Geometry check sheet. Reference: drawing and pictorial views, mm from the part's lowest x, y, z. A direction names the side the tool comes from. Give positions to 0.01 mm unless a question says otherwise; leave off trailing zeros. Write each loop counter-clockwise with the first axis right and the second up, starting at its lowest first coordinate (ties: lowest second). Pieces come first, ordered by that corner, then holes. Notation, with made-up numbers: (-0.75, 54.5) -> (51.25, 54.5) arc R3 cw to (51.25, 59.5) -> close; hole circle Ø2 at (12, -5). An arc over 180 degrees is marked (long way). Answer as CSV lines item,"result".
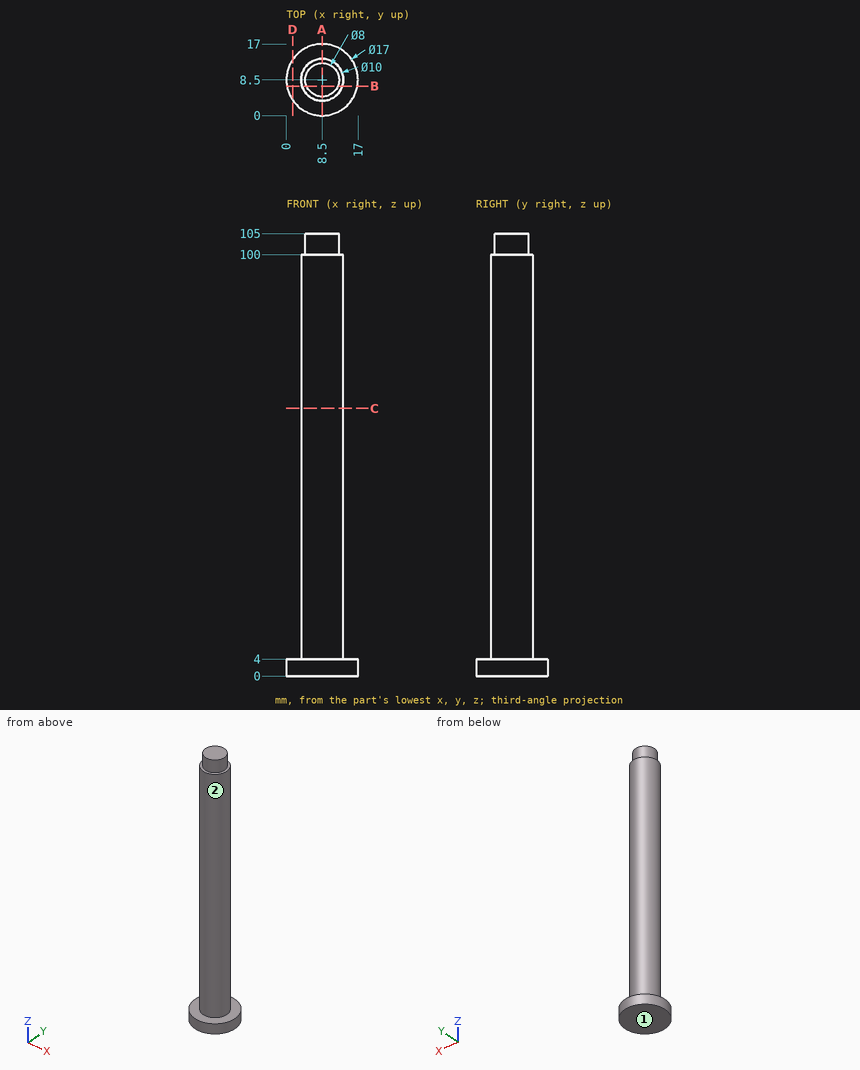
1) Section check C-C (z = 63.5). Record the boundary of the cut face in (x, y), and give its area (3 significant figures).
Reported:
outline,"circle Ø10 at (8.5, 8.5)"
area,"78.5 mm²"
2) Scan lines: line 1 along Y through (x, z) = (11.5, 61); line 2 along Y through (x, z) = (8.5, 78); line 3 along Z through (x, y) = (3, 6.25). Record each from-to range of solid material in increasing order.
Reported:
line 1,"4.5 to 12.5"
line 2,"3.5 to 13.5"
line 3,"0 to 4"
3) Section check D-D (x = 1.5). Record the boundary of the cut face in (y, z).
Reported:
outline,"(3.68, 0) -> (13.32, 0) -> (13.32, 4) -> (3.68, 4) -> close"
4) Section check A-A (x = 8.5). Record the boundary of the cut face in (y, z).
Reported:
outline,"(0, 0) -> (17, 0) -> (17, 4) -> (13.5, 4) -> (13.5, 100) -> (12.5, 100) -> (12.5, 105) -> (4.5, 105) -> (4.5, 100) -> (3.5, 100) -> (3.5, 4) -> (0, 4) -> close"
5) Depth check by flat-ended pin: pin 1 (1.5 mm diameter, centred on x = 6, y = 14.5, fed in from +Z); pin 2 (1 mm diameter, centred on y = 12, z = 92.5, fed in from -X); pin 3 (6 mm diameter, centred on y = 4, z = 67.5, fed in from +X). Enter the tip coordinate at first touch or a pass-through.
Reported:
pin 1,"z = 4"
pin 2,"x = 4.5"
pin 3,"x = 13.27"
6) Tool access check on the marked faces 1 and 2. Record the directions out of +Z, -Z, +X, -X, +Y, -Y that give a thin tool (end or side, any length) a straight path to the whole face; none if there is none.
Reported:
face 1,"-Z, +X, -X, +Y, -Y"
face 2,"+Z"
7) Section check B-B (y = 7). Record the boundary of the cut face in (x, z), and give its area (3 significant figures).
Reported:
outline,"(0.13, 0) -> (16.87, 0) -> (16.87, 4) -> (13.27, 4) -> (13.27, 100) -> (12.21, 100) -> (12.21, 105) -> (4.79, 105) -> (4.79, 100) -> (3.73, 100) -> (3.73, 4) -> (0.13, 4) -> close"
area,"1,020 mm²"
